```python
from build123d import *

# Parameters (mm, degrees)
BOSS_EXTRUDE1_DEPTH     = 6.35
SKETCH1_4_W             = 3.683
SKETCH1_4_H             = 17.441333418
CUT_EXTRUDE2_DEPTH      = 7.35
CUT_EXTRUDE2_DEPTH_BACK = 7.35
SKETCH1_3_W             = 6.477
SKETCH1_3_H             = 6.35
BOSS_EXTRUDE2_DEPTH     = 1.524
SKETCH2_R               = 1.5875
CUT_EXTRUDE1_DEPTH      = 51.8
FILLET1_R               = 4.826
FILLET2_R               = 6.35
SKETCH3_W               = 1.27
SKETCH3_H               = 9.525
CUT_EXTRUDE3_DEPTH      = 7.35
CUT_EXTRUDE3_DEPTH_BACK = 7.35
SKETCH4_W               = 4.826
SKETCH4_H               = 33.0835
CUT_EXTRUDE5_DEPTH      = 47.625
SKETCH5_W               = 3.683
SKETCH5_H               = 6.096
CUT_EXTRUDE6_DEPTH      = 4.826
CUT_EXTRUDE7_START      = -12.7
SKETCH5_2_W             = 3.683
SKETCH5_2_H             = 6.096
CUT_EXTRUDE7_DEPTH      = 4.826


with BuildPart() as part:
    # Sketch1 → Boss-Extrude1 (new body, symmetric)
    with BuildSketch(Plane(origin=(0, 0, 0), x_dir=(0, 0, -1), z_dir=(1, 0, 0))):
        Polygon((-19.939, 3.175), (-19.939, 0), (19.939, 0), (19.939, 50.8), (13.1445, 50.8), (13.1445, 35.729333418), (-5.167312548, 3.175), align=None)
    extrude(amount=BOSS_EXTRUDE1_DEPTH, both=True)

    # Sketch1<4> → Cut-Extrude2 (cut, two sides)
    with BuildSketch(Plane(origin=(0, 0, 0), x_dir=(0, 0, -1), z_dir=(1, 0, 0))) as cut_extrude2_sk:
        with Locations((11.303, 14.816666709)):
            Rectangle(SKETCH1_4_W, SKETCH1_4_H)
    extrude(amount=CUT_EXTRUDE2_DEPTH, mode=Mode.SUBTRACT)
    extrude(cut_extrude2_sk.sketch, amount=-CUT_EXTRUDE2_DEPTH_BACK, mode=Mode.SUBTRACT)

    # Sketch1<3> → Boss-Extrude2 (add, symmetric)
    with BuildSketch(Plane(origin=(0, 0, 0), x_dir=(0, 0, -1), z_dir=(1, 0, 0))):
        Polygon((13.1445, 0), (12.065, 0), (12.065, -6.35), (19.939, -6.35), (19.939, 0), align=None)
        with Locations((2.4765, -3.175)):
            Rectangle(SKETCH1_3_W, SKETCH1_3_H)
    extrude(amount=BOSS_EXTRUDE2_DEPTH, both=True)

    # Sketch2 → Cut-Extrude1 (cut, through all)
    with BuildSketch(Plane.XZ):
        with Locations((0, 15.1765)):
            Circle(SKETCH2_R)
    extrude(amount=-CUT_EXTRUDE1_DEPTH, mode=Mode.SUBTRACT)

    # Fillet1
    fillet1_edges = [part.edges().sort_by_distance(p)[0] for p in [
        (-6.35, 25.4, -19.939),
        (6.35, 25.4, -19.939),
    ]]
    fillet(fillet1_edges, radius=FILLET1_R)

    # Fillet2
    fillet2_edges = [part.edges().sort_by_distance(p)[0] for p in [
        (0, 3.175, 5.167312548),
    ]]
    fillet(fillet2_edges, radius=FILLET2_R)

    # Sketch3 → Cut-Extrude3 (cut, two sides)
    with BuildSketch(Plane(origin=(0, 0, 0), x_dir=(0, 0, -1), z_dir=(1, 0, 0))) as cut_extrude3_sk:
        with Locations((19.304, 33.3375)):
            Rectangle(SKETCH3_W, SKETCH3_H)
    extrude(amount=CUT_EXTRUDE3_DEPTH, mode=Mode.SUBTRACT)
    extrude(cut_extrude3_sk.sketch, amount=-CUT_EXTRUDE3_DEPTH_BACK, mode=Mode.SUBTRACT)

    # Sketch4 → Cut-Extrude5 (cut)
    with BuildSketch(Plane(origin=(0, 50.8, 0), x_dir=(1, 0, 0), z_dir=(0, 1, 0))):
        with Locations((-3.937, -3.39725)):
            Rectangle(SKETCH4_W, SKETCH4_H)
        with Locations((3.937, -3.39725)):
            Rectangle(SKETCH4_W, SKETCH4_H)
    extrude(amount=-CUT_EXTRUDE5_DEPTH, mode=Mode.SUBTRACT)

    # Sketch5 → Cut-Extrude6 (cut)
    with BuildSketch(Plane(origin=(6.35, 0, 0), x_dir=(0, 0, -1), z_dir=(1, 0, 0))):
        with Locations((11.303, 3.048)):
            Rectangle(SKETCH5_W, SKETCH5_H)
    extrude(amount=-CUT_EXTRUDE6_DEPTH, mode=Mode.SUBTRACT)

    # Sketch5<2> → Cut-Extrude7 (cut)
    with BuildSketch(Plane(origin=(6.35, 0, 0), x_dir=(0, 0, -1), z_dir=(1, 0, 0)).offset(CUT_EXTRUDE7_START)):
        with Locations((11.303, 3.048)):
            Rectangle(SKETCH5_2_W, SKETCH5_2_H)
    extrude(amount=CUT_EXTRUDE7_DEPTH, mode=Mode.SUBTRACT)


solid = part.part
```
Part model, mm, in its own coordinate system. A direction names the side the tool comes from. Coordinates: 2 decimals unless noted, no trailing zeros. Loops run counter-clockwise (first coordinate to the right, second up) from the corner with the lowest first, then second, coordinate; pieces in that order, holes last. Notation, with made-up numbers: (56, 86) - (68, 86) arc R22 cw to (68, 120) - close; hole circle Ø6 at (-11, 84.25). An arc over 180 degrees is marked (long way). Write item = value, one per line. Start each with the question number.
Item 1: Cut at A-A, the plane x = 0. State how many separate pieces and enclosed holes the cut face has, and give its area (3 significant figures).
Item 2: Flat gauge pins, fed straight in: pin 1 Ø1.4 at (x, z) = (-5, -18) entering from -Y; pin 2 Ø1.9 at (y, z) = (-3.5, -2) entering from -X; pin 3 Ø1.6 at (x, y) = (3, 1.5) entering from -Z. Where does each tip first touch, or does it go through?
Item 3: Mould opens along Z. For faces 1 (the flat face through (0, 6.096, -11)), 2 (the flat face through (0, 11, -19.939)), 3 (the flat face through (0, -3, 0.762)) say: released by +Z, released by -Z, zero draft, split by the parting line, or undercut.
Item 4: Cut at B-B, the plane y = 12. Give the cut face in (x, z).
Item 5: Wall check: L1, parallel to Z at x = 0, y = 2.4; L2, parallel to Z at x = 2.25, y = 31; L3, parallel to Y at x = 3.25, z = 12 (3 decimals). Give the ranges that are in metal, low to high. Write a range as from..to.
Item 6: Cut at D-D, the plane x = 3. Give the cut face in (y, z) (1 decimal), and give its area (3 significant figures).
Item 7: Cut at C-C, the plane z = -14.5. Give the cut face in (x, y), and give its area (3 significant figures).
Item 8: 3-axis set-ups, long thin cutter, end or side, ignore diameter. For faces 4 (the flat face through (3, 3.175, 5)), 5 (the flat face through (3, 26, -13.144)), 6 (the flat face through (0, -3, -12.065)): which of +Z, -Z, +X, -X, +Y, -Y reach the whole face in a straight line?
The answers:
q1.separate_pieces = 2
q1.enclosed_holes = 1
q1.area = 755 mm2
q2.pin_1 = 0
q2.pin_2 = -1.52
q2.pin_3 = -19.89
q3.face_1 = undercut
q3.face_2 = released by -Z
q3.face_3 = released by +Z
q4.outline = (-6.35, -15.11) arc R4.83 ccw to (-1.52, -19.94) - (1.52, -19.94) arc R4.83 ccw to (6.35, -15.11) - (6.35, -13.14) - (-6.35, -13.14) - close; (-1.52, -9.46) - (1.52, -9.46) - (1.52, 0.2) - (-1.52, 0.2) - close
q5.L1 = -19.94..13.59, 16.76..19.94
q5.L2 = -18.67..-13.14
q5.L3 = 0..3.175
q6.outline = (0, -19.7) - (28.6, -19.7) - (28.6, -18.7) - (38.1, -18.7) - (38.1, -19.7) - (50.8, -19.7) - (50.8, -13.1) - (0, -13.1) - close; (0, -9.5) - (3.2, -9.5) - (3.2, 19.9) - (0, 19.9) - close
q6.area = 417 mm2
q7.outline = (-6.35, 0) - (-1.52, 0) - (-1.52, -6.35) - (1.52, -6.35) - (1.52, 0) - (6.35, 0) - (6.35, 50.8) - (-6.35, 50.8) - close
q7.area = 665 mm2
q8.face_4 = +Z, +Y
q8.face_5 = none
q8.face_6 = +X, -X, -Y
